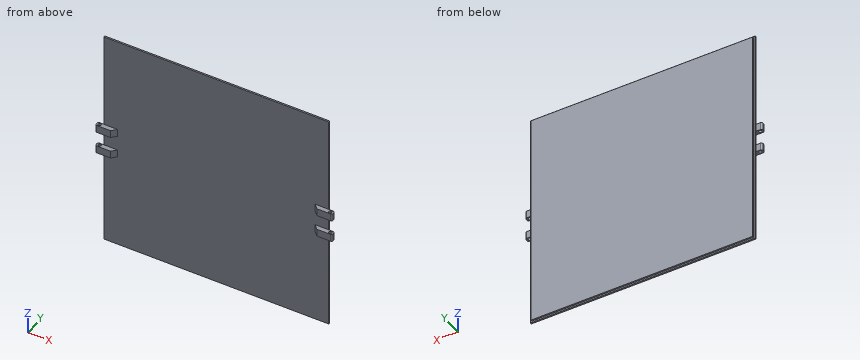
```python
from build123d import *

# Parameters (mm, degrees)
SKETCH1_R           = 10
SKETCH1_R_2         = 7.5
BOSS_EXTRUDE1_DEPTH = 25
THREAD1_PITCH       = 0.3175
SKETCH4_W           = 146
SKETCH4_H           = 146
BOSS_EXTRUDE2_DEPTH = 2
SKETCH5_W           = 148
SKETCH5_H           = 148
BOSS_EXTRUDE3_DEPTH = 1
BOSS_EXTRUDE4_START = 7.5
SKETCH6_W           = 10
SKETCH6_H           = 3
SKETCH6_R           = 1
BOSS_EXTRUDE4_DEPTH = 2.5
BOSS_EXTRUDE5_START = -7.5
SKETCH6_2_W         = 10
SKETCH6_2_H         = 3
SKETCH6_2_R         = 1
BOSS_EXTRUDE5_DEPTH = 2.5
SKETCH9_R           = 18.995637602
CUT_EXTRUDE1_DEPTH  = 111.385687501
CHAMFER1_SIZE       = 3
FILLET1_R           = 1


with BuildPart() as part:
    # Sketch1 → Boss-Extrude1 (new body)
    with BuildSketch(Plane(origin=(0, 0, 0), x_dir=(1, 0, 0), z_dir=(0, 1, 0))):
        with Locations(Location((0, 0, 0), (0, 0, 270))):
            Circle(SKETCH1_R)
        with Locations(Location((0, 0, 0), (0, 0, 270))):
            Circle(SKETCH1_R_2, mode=Mode.SUBTRACT)
    extrude(amount=BOSS_EXTRUDE1_DEPTH)

    # Thread1: the profile of Thread Profile1 profile screwed along a right-hand helix of 18.897638 turns, 6 arcs to a turn; built about Z, then put on its axis
    thread1_z = Axis((0, 0, 0), (0, 0, 1))
    thread1_corners = [(10.0003, 0, -0.000173205), (10.0003, 0, 0.277985704), (9.828148085, 0, 0.17859375), (9.828148085, 0, 0.09921875)]
    with BuildLine(mode=Mode.PRIVATE) as thread1_profile:
        Line(thread1_corners[0], thread1_corners[1])
        Line(thread1_corners[1], thread1_corners[2])
        Line(thread1_corners[2], thread1_corners[3])
        Line(thread1_corners[3], thread1_corners[0])
    thread1_cap = Face(thread1_profile.wire())
    thread1_turn_angles = [0, 30, 60, 90, 120, 150, 180, 210, 240, 270, 300, 330, 360]
    thread1_turn_weights = [1, 0.8660254037844387, 1, 0.8660254037844387, 1, 0.8660254037844387, 1, 0.8660254037844387, 1, 0.8660254037844387, 1, 0.8660254037844387, 1]
    thread1_turn_rails = [Edge.make_bspline([Vector(p[0], p[1], 0).rotate(thread1_z, thread1_turn_angles[k]) / thread1_turn_weights[k] + Vector(0, 0, p[2] + THREAD1_PITCH * thread1_turn_angles[k] / 360) for k in range(13)], [0, 0, 0, 1, 1, 2, 2, 3, 3, 4, 4, 5, 5, 6, 6, 6], 2, thread1_turn_weights) for p in thread1_corners]
    thread1_turn_sides = [Face.make_surface_from_curves(thread1_turn_rails[p[0]], thread1_turn_rails[p[1]]) for p in [(0, 1), (1, 2), (2, 3), (3, 0)]]
    thread1_last_angles = [6480, 6510, 6540, 6570, 6600, 6630, 6660, 6690, 6720, 6750, 6780, 6791.57480315, 6803.149606299]
    thread1_last_weights = [1, 0.8660254037844387, 1, 0.8660254037844387, 1, 0.8660254037844387, 1, 0.8660254037844387, 1, 0.8660254037844387, 1, 0.9796635825089068, 1]
    thread1_last_rails = [Edge.make_bspline([Vector(p[0], p[1], 0).rotate(thread1_z, thread1_last_angles[k]) / thread1_last_weights[k] + Vector(0, 0, p[2] + THREAD1_PITCH * thread1_last_angles[k] / 360) for k in range(13)], [0, 0, 0, 1, 1, 2, 2, 3, 3, 4, 4, 5, 5, 6, 6, 6], 2, thread1_last_weights) for p in thread1_corners]
    thread1_last_sides = [Face.make_surface_from_curves(thread1_last_rails[p[0]], thread1_last_rails[p[1]]) for p in [(0, 1), (1, 2), (2, 3), (3, 0)]]
    thread1 = Plane(origin=(0, -0.5, 0), x_dir=(1, 0, 0), z_dir=(0, 1, 0)) * Solid(Shell([*[p.moved(Location((0, 0, THREAD1_PITCH * i))) for i in range(18) for p in thread1_turn_sides], *thread1_last_sides, thread1_cap, thread1_cap.rotate(thread1_z, 6803.149606299).moved(Location((0, 0, THREAD1_PITCH * 6803.149606299 / 360)))]))
    add(thread1, mode=Mode.SUBTRACT)

    # Sketch4 → Boss-Extrude2 (add)
    with BuildSketch(Plane(origin=(0, 25, 0), x_dir=(1, 0, 0), z_dir=(0, 1, 0))):
        Rectangle(SKETCH4_W, SKETCH4_H)
    extrude(amount=BOSS_EXTRUDE2_DEPTH)

    # Sketch5 → Boss-Extrude3 (add)
    with BuildSketch(Plane.XZ.offset(-25)):
        Rectangle(SKETCH5_W, SKETCH5_H)
    extrude(amount=-BOSS_EXTRUDE3_DEPTH)

    # Sketch6 → Boss-Extrude4 (add, symmetric)
    # profile 1 of 2: a face of its own
    with BuildSketch(Plane.XY.offset(BOSS_EXTRUDE4_START)):
        with Locations((73, 23.5)):
            Rectangle(SKETCH6_W, SKETCH6_H)
        with Locations((76, 23.5)):
            Circle(SKETCH6_R, mode=Mode.SUBTRACT)
    # profile 2 of 2: a face of its own
    with BuildSketch(Plane.XY.offset(BOSS_EXTRUDE4_START)):
        with Locations((-73, 23.5)):
            Rectangle(SKETCH6_W, SKETCH6_H)
        with Locations(Location((-76, 23.5, 0), (0, 0, 180))):
            Circle(SKETCH6_R, mode=Mode.SUBTRACT)
    extrude(amount=BOSS_EXTRUDE4_DEPTH, both=True)

    # Sketch6<2> → Boss-Extrude5 (add, symmetric)
    # profile 1 of 2: a face of its own
    with BuildSketch(Plane.XY.offset(BOSS_EXTRUDE5_START)):
        with Locations((73, 23.5)):
            Rectangle(SKETCH6_2_W, SKETCH6_2_H)
        with Locations((76, 23.5)):
            Circle(SKETCH6_2_R, mode=Mode.SUBTRACT)
    # profile 2 of 2: a face of its own
    with BuildSketch(Plane.XY.offset(BOSS_EXTRUDE5_START)):
        with Locations((-73, 23.5)):
            Rectangle(SKETCH6_2_W, SKETCH6_2_H)
        with Locations(Location((-76, 23.5, 0), (0, 0, 180))):
            Circle(SKETCH6_2_R, mode=Mode.SUBTRACT)
    extrude(amount=BOSS_EXTRUDE5_DEPTH, both=True)

    # Sketch9 → Cut-Extrude1 (cut, through all)
    with BuildSketch(Plane.XZ.offset(-25)):
        Circle(SKETCH9_R)
    extrude(amount=CUT_EXTRUDE1_DEPTH, mode=Mode.SUBTRACT)

    # Chamfer1
    chamfer1_edges = [part.edges().sort_by_distance(p)[0] for p in [
        (68, 25, -7.5),
        (68, 25, 7.5),
        (-68, 25, -7.5),
        (-68, 25, 7.5),
    ]]
    chamfer(chamfer1_edges, length=CHAMFER1_SIZE - 0.0001)  # a hair under: the kernel refuses the full size

    # Fillet1
    fillet1_edges = [part.edges().sort_by_distance(p)[0] for p in [
        (78, 22, -7.5),
        (78, 25, -7.5),
        (-78, 25, -7.5),
        (-78, 22, -7.5),
        (78, 22, 7.5),
        (78, 25, 7.5),
        (-78, 25, 7.5),
        (-78, 22, 7.5),
    ]]
    fillet(fillet1_edges, radius=FILLET1_R)


solid = part.part
```
Design review of the part built by this model. Coordinates are the model's own, in mm. Round coordinates to 2 decimals unless told otherwise and drop trailing zeros. Order: outer loops, then holes, each group sorted by start corner. A loop starts at its lowest first (then second) coordinate and runs counter-clockwise, first axis right, second up. Notation, with made-up numbers: (71.5, 73.5) - (112.5, 73.5) arc R11 cw to (112.5, 94.5) - close; hole circle Ø3 at (37.25, -22.5). An arc over 180 degrees is marked (long way). One line per question, with ' | ' between items.
Item 1: Take a section at B-B, the plane z = 52. Write out the cut boundary in (x, y), then the cut area to 3 significant figures.
Checks:
outline: (-74, 25) - (74, 25) - (74, 26) - (73, 26) - (73, 27) - (-73, 27) - (-73, 26) - (-74, 26) - close | area: 294 mm²
Item 2: Take a section at A-A, the plane x = -7. Write out the cut boundary in (y, z), then the cut area to 3 significant figures.
Checks:
outline: (25, -74) - (26, -74) - (26, -73) - (27, -73) - (27, 73) - (26, 73) - (26, 74) - (25, 74) - close | area: 294 mm²
Item 3: For P1, Ø1.5, axis at x = 68.5, y = 23.5, coming from the -Z side; P2, Ø0.8, axis at x = 19.5, y = 26.5, coming from the +Z side; P3, Ø2.5, axis at x = 69.5, y = 23, coming from the +Z side, all flat-tipped, find the tip position at first contact; note any pin that passes through.
Checks:
P1: z = -10 | P2: z = 73 | P3: z = 10
Item 4: Wall thickness on line 1 (Y direction, x = 76, z = 6.6); line 2 (X direction, y = 24.25, z = 6); line 3 (X direction, y = 26.25, z = 48.5): over which ranges is each line inside the solid? List them lowest first. Write a range as [from, to].
Checks:
line 1: [22, 22.5], [24.5, 25] | line 2: [-77.97, -76.66], [-75.34, -65.75], [65.75, 75.34], [76.66, 77.97] | line 3: [-73, 73]
